Could you check a few things on this model? Use its own coordinates, in mm. Face numbers are marked on the shaded views. Coordinates: 2 decimals unless noted, no trailing zeros. Write each loop counter-clockwise with the first axis right and the second up, starting at its lowest first coordinate (ties: lowest second). Pieces come first, ordered by that corner, then holes.
Item 1: I want a section at D-D on y = 57. Please give me the cut outline in (x, z) (3 decimals), then the cut area to 3 significant figures.
Item 2: Thinking about a two-plate mould opening in Y: for the marked faces 1, 2, 3 and 4, which applies, +Y half, -Y half, draft (parallel to the pull), parting line (faces both ways), or undercut?
Item 3: I want a section at A-A on z = 0. Please give me the cut outline in (x, y) (3 decimals).
Item 4: I want a section at C-C on y = 40.25. Please give me the cut outline in (x, z) (3 decimals).
Item 5: For P1, Ø3, axis at x = 0, y = 40.25, coming from the -Z side; P2, Ø1, axis at y = 20, z = -3.5, coming from the +X side; P3, Ø10, axis at y = 36.5, z = 4.5, coming from the +X side; P4, Ø3, axis at x = -5.5, y = 50, coming from the -Z side, each with a flat end and sliding along its axis, tell me the tip position at first contact or that it passes through.
Item 6: If I drill on probe 1 along Y at (x, z) = (0, -7.65); probe 2 along Z at (x, y) = (-3.5, 40.25); probe 3 along Y at (x, z) = (1.5, 0), over which ranges is the centre line in solid material (lowest first)?
Item 7: I want a section at B-B on x = 0. Please give me the cut outline in (y, z) (3 decimals).
from build123d import *

# Parameters (mm, degrees)
SKETCH1_R               = 8.495
BOSS_EXTRUDE1_DEPTH     = 80.5
CHAMFER1_SIZE           = 0.75
CUT_EXTRUDE1_DEPTH      = 82.391523207
CUT_EXTRUDE1_DEPTH_BACK = 82.391523207
SKETCH2_R               = 7.5
CUT_EXTRUDE2_DEPTH      = 82.391523228
CUT_EXTRUDE2_DEPTH_BACK = 82.391523228
SKETCH3_R               = 2.5


with BuildPart() as part:
    # Sketch1 → Boss-Extrude1 (new body)
    with BuildSketch(Plane(origin=(0, 0, 0), x_dir=(1, 0, 0), z_dir=(0, 1, 0))):
        with Locations(Location((0, 0, 0), (0, 0, 270))):
            Circle(SKETCH1_R)
    extrude(amount=BOSS_EXTRUDE1_DEPTH)

    # Chamfer1
    chamfer1_edges = [part.edges().sort_by_distance(p)[0] for p in [
        (0, 0, -8.495),
        (0, 80.5, -8.495),
    ]]
    chamfer(chamfer1_edges, length=CHAMFER1_SIZE)

    # Sketch2 → Cut-Extrude1 (cut, two sides: drawn at the far end of the back side and taken through both)
    with BuildSketch(Plane(origin=(0, 0, 0), x_dir=(0, 0, -1), z_dir=(1, 0, 0)).offset(-CUT_EXTRUDE1_DEPTH_BACK)):
        with Locations((0, 40.25)):
            Circle(SKETCH2_R)
    extrude(amount=CUT_EXTRUDE1_DEPTH + CUT_EXTRUDE1_DEPTH_BACK, mode=Mode.SUBTRACT)

    # Sketch3 → Cut-Extrude2 (cut, two sides: drawn at the far end of the back side and taken through both)
    with BuildSketch(Plane.XY.offset(-CUT_EXTRUDE2_DEPTH_BACK)):
        with Locations((0, 40.25)):
            Circle(SKETCH3_R)
    extrude(amount=CUT_EXTRUDE2_DEPTH + CUT_EXTRUDE2_DEPTH_BACK, mode=Mode.SUBTRACT)


solid = part.part
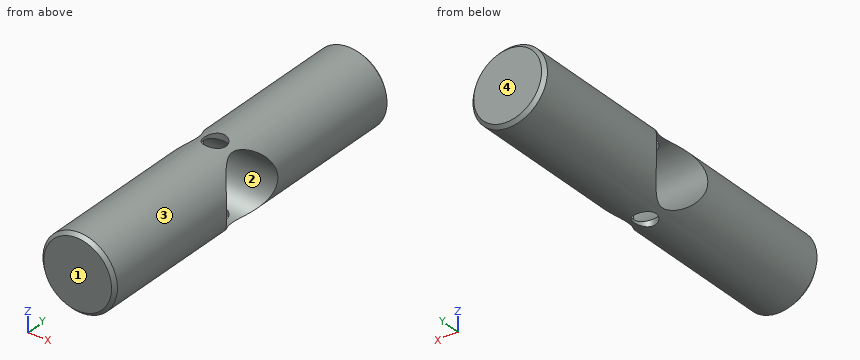
Response values:
1. outline: circle Ø16.99 at (0, 0)
1. area: 227 mm2
2. face 1: -Y half
2. face 2: undercut
2. face 3: draft
2. face 4: +Y half
3. outline: (-8.495, 0.75) - (-7.745, 0) - (7.745, 0) - (8.495, 0.75) - (8.495, 32.75) - (-8.495, 32.75) - close; (-8.495, 47.75) - (8.495, 47.75) - (8.495, 79.75) - (7.745, 80.5) - (-7.745, 80.5) - (-8.495, 79.75) - close
4. outline: (-3.989, -7.5) arc R8.495 ccw to (-2.5, -8.119) - (-2.5, -7.5) - close; (-3.989, 7.5) - (-2.5, 7.5) - (-2.5, 8.119) arc R8.495 ccw to start; (2.5, -8.119) arc R8.495 ccw to (3.989, -7.5) - (2.5, -7.5) - close; (2.5, 7.5) - (3.989, 7.5) arc R8.495 ccw to (2.5, 8.119) - close
5. P1: passes through
5. P2: stops at x = 7.95
5. P3: stops at x = 8.42
5. P4: stops at z = -7.49
6. probe 1: y = 0 to 37.75, 42.75 to 80.5
6. probe 2: z = -7.74 to -7.5, 7.5 to 7.74
6. probe 3: y = 0 to 32.75, 47.75 to 80.5
7. outline: (0, -7.745) - (0.75, -8.495) - (37.75, -8.495) - (37.75, -7.071) arc R7.5 cw to (37.75, 7.071) - (37.75, 8.495) - (0.75, 8.495) - (0, 7.745) - close; (42.75, -8.495) - (79.75, -8.495) - (80.5, -7.745) - (80.5, 7.745) - (79.75, 8.495) - (42.75, 8.495) - (42.75, 7.071) arc R7.5 cw to (42.75, -7.071) - close
